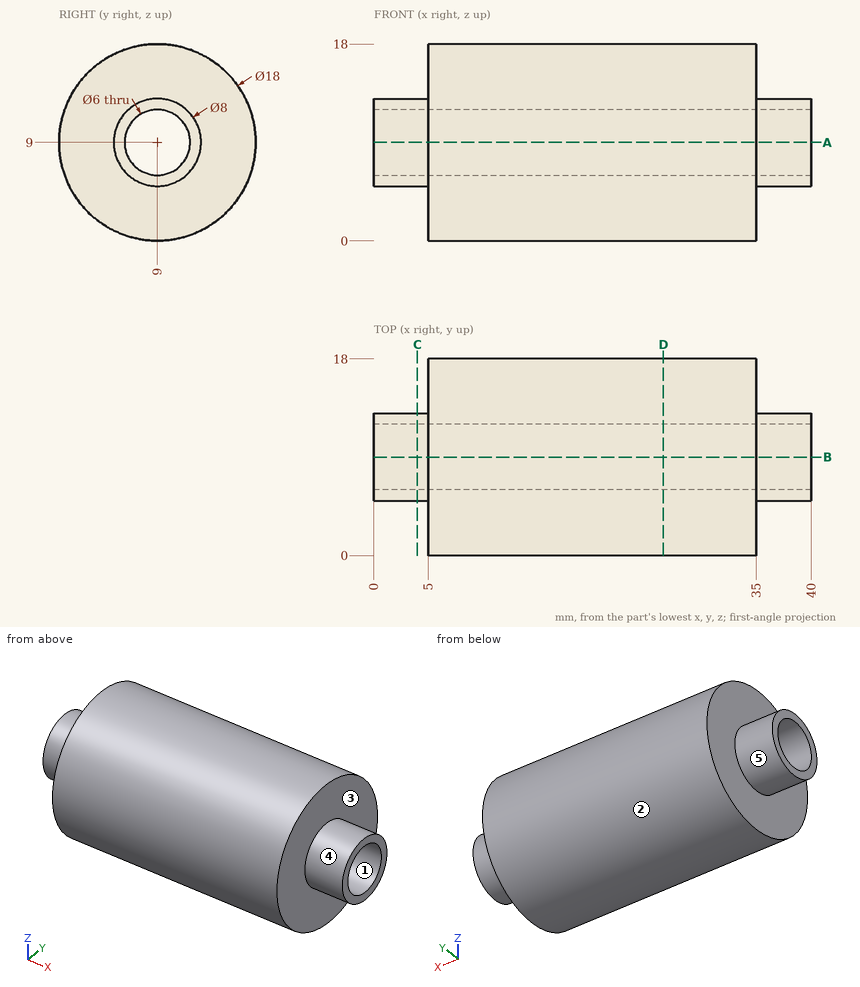
Design review of the part shown in the three views and the two pictorial views. Dimensions are in mm from the part's minimum x, y and z. A direction names the side the tool comes from. Round coordinates to 2 decimals unless told otherwise and drop trailing zeros. Loops run counter-clockwise (first coordinate to the right, second up) from the corner with the lowest first, then second, coordinate; pieces in that order, holes last. Notation, with made-up numbers: (-21, -3.5) - (12, -3.5) arc R4 cw to (12, 1.5) - close; hole circle Ø9 at (-1, -21). An arc over 180 degrees is marked (long way). Use CSV: the item, a comma, the result in double quotes.
(1) For line 1 (Y direction, x = 18, z = 9); line 2 (X direction, y = 7.5, z = 14); line 3 (Z direction, x = 21.5, y = 11), list the stretches that pass through material, from the lowest coordinate up.
Working result:
line 1,"y = 0 to 6, 12 to 18"
line 2,"x = 5 to 35"
line 3,"z = 0.23 to 6.76, 11.24 to 17.77"
(2) Machinability: for the marked faces 4 and 5, which of the approach directions +Z, -Z, +X, -X, +Y, -Y give a long, thin tool a straight path to every point of the face, cutting with its end or side? Answer none if there is none.
Working result:
face 4,"+X"
face 5,"-X"
(3) Clearance check with flat-ended pins moving along their axes: P1, Ø10, axis at y = 14.5, z = 7.5, coming from the -X side; P2, Ø2, axis at y = 10.5, z = 15.5, coming from the +X side; P3, Ø1.5, axis at x = 29, y = 2.5, coming from the +Z side; P4, Ø5, axis at y = 9, z = 9, coming from the +X side. State where each tip first meets the part, or that it passes through.
Working result:
P1,"stops at x = 0"
P2,"stops at x = 35"
P3,"stops at z = 15.92"
P4,"passes through"
(4) Take a section at A-A, the plane z = 9. Give the boundary of the cut face in (x, y).
Working result:
outline,"(0, 5) - (5, 5) - (5, 0) - (35, 0) - (35, 5) - (40, 5) - (40, 6) - (0, 6) - close; (0, 12) - (40, 12) - (40, 13) - (35, 13) - (35, 18) - (5, 18) - (5, 13) - (0, 13) - close"
(5) Take a section at D-D, the plane x = 26.5. Give the boundary of the cut face in (y, z), plus the area to 3 significant figures.
Working result:
outline,"circle Ø18 at (9, 9); hole circle Ø6 at (9, 9)"
area,"226 mm^2"
(6) The part is to be moulded in two halves that separate along Y. For the marked faces 1, 2 and 3, say which applies: pulls with the +Y half, pulls with the -Y half, needs draft (parallel to the pull), parting line crosses it, or undercut.
Working result:
face 1,"undercut"
face 2,"parting line crosses it"
face 3,"needs draft"
(7) Take a section at C-C, the plane x = 4. Give the boundary of the cut face in (y, z).
Working result:
outline,"circle Ø8 at (9, 9); hole circle Ø6 at (9, 9)"
